from build123d import *

# Parameters (mm, degrees)
SKETCH1_R             = 75
BOSS_EXTRUDE1_DEPTH   = 10
SKETCH2_R             = 59.5
BOSS_EXTRUDE2_DEPTH   = 240
BOSS_EXTRUDE3_DEPTH   = 30
SKETCH7_R             = 10
CUT_EXTRUDE1_DEPTH    = 30
SKETCH9_R             = 4.5
CUT_EXTRUDE3_DEPTH    = 10
BODY_MOVE_COPY1_ANGLE = 90


with BuildPart() as part:
    # Sketch1 → Boss-Extrude1 (new body)
    with BuildSketch(Plane(origin=(0, 0, 0), x_dir=(1, 0, 0), z_dir=(0, 1, 0))):
        Circle(SKETCH1_R)
    extrude(amount=BOSS_EXTRUDE1_DEPTH)

    # Sketch2 → Boss-Extrude2 (add)
    with BuildSketch(Plane(origin=(0, 10, 0), x_dir=(1, 0, 0), z_dir=(0, 1, 0))):
        Circle(SKETCH2_R)
    extrude(amount=BOSS_EXTRUDE2_DEPTH)

    # Sketch6 → Boss-Extrude3 (add)
    with BuildSketch(Plane(origin=(0, 250, 0), x_dir=(1, 0, 0), z_dir=(0, 1, 0))):
        with BuildLine():
            Line((48.117044797, 35), (80, 35))
            ThreePointArc((80, 35), (101.213203436, 26.213203436), (110, 5))
            Line((110, 5), (110, -5))
            ThreePointArc((110, -5), (101.213203436, -26.213203436), (80, -35))
            Line((80, -35), (48.117044797, -35))
            ThreePointArc((48.117044797, -35), (59.5, 0), (48.117044797, 35))
        make_face()
    extrude(amount=-BOSS_EXTRUDE3_DEPTH)

    # Sketch7 → Cut-Extrude1 (cut)
    with BuildSketch(Plane(origin=(0, 250, 0), x_dir=(1, 0, 0), z_dir=(0, 1, 0))):
        Circle(SKETCH7_R)
    extrude(amount=-CUT_EXTRUDE1_DEPTH, mode=Mode.SUBTRACT)

    # Sketch9 → Cut-Extrude3 (cut)
    with BuildSketch(Plane(origin=(0, 10, 0), x_dir=(1, 0, 0), z_dir=(0, 1, 0))):
        with Locations((0, 67.096454414)):
            Circle(SKETCH9_R)
        with Locations((-67.440146023, 0)):
            Circle(SKETCH9_R)
    cut_extrude3 = extrude(amount=-CUT_EXTRUDE3_DEPTH, mode=Mode.SUBTRACT)

    # Mirror2: Cut-Extrude3 across plane
    add(cut_extrude3.mirror(Plane.XY), mode=Mode.SUBTRACT)

    # Mirror3: Cut-Extrude3 across plane
    add(cut_extrude3.mirror(Plane(origin=(0, 0, 0), x_dir=(0, 0, 1), z_dir=(1, 0, 0))), mode=Mode.SUBTRACT)


with BuildPart() as part_1:
    # Body-Move/Copy1: moved
    add(part.part.rotate(Axis((0, 0, 0), (1, 0, 0)), BODY_MOVE_COPY1_ANGLE))


solid = part_1.part
Work out the finished part from the listing and answer in its coordinate system (mm). A direction names the side the tool comes from. Coordinates: 2 decimals unless noted, no trailing zeros. Write each loop counter-clockwise with the first axis right and the second up, starting at its lowest first coordinate (ties: lowest second). Pieces come first, ordered by that corner, then holes.
1. Flat-ended cylindrical pins translate along their axes: pin 1 (10.5 mm diameter, centred on x = 0, y = 67.1, fed in from +Z); pin 2 (15 mm diameter, centred on x = 63.5, z = 228, fed in from +Y); pin 3 (7 mm diameter, centred on x = 67.44, y = 0, fed in from -Z); pin 4 (11.5 mm diameter, centred on x = 0, y = -67.1, fed in from -Z). Find the tip coordinate at first contact, or state that the pin passes through.
Results list:
pin 1: stops at z = 10
pin 2: stops at y = 35
pin 3: stops at z = 220
pin 4: stops at z = 0
2. For a pull along Y with two mould halves and no side action, classify faces 6 (the cylindrical face through (100.979, 26.445, 235.21)), 7 (the flat face through (79, 0, 220)), 8 (the cylindrical face through (-2.17, -9.76, 235.21)), 9 (the cylindrical face through (2.42, -70.89, 5.07)) as +Y half, -Y half, draft (parallel to the pull), parting line (faces both ways), or undercut.
Results list:
face 6: +Y half
face 7: draft
face 8: undercut
face 9: undercut
3. For faces 1 (the flat face through (64, 35, 235)), 2 (the flat face through (0, 0, 220)), 3 (the flat face through (64, -35, 235)), 4 (the flat face through (-34, -50, 10)), 5 (the cylindrical face through (-9.764, 74.362, 4.93)), determine the directions among +Z, -Z, +X, -X, +Y, -Y from which every point of the face is accessible in a straight line to the end or side of a thin tool.
Results list:
face 1: +Z, +X, +Y
face 2: +Z
face 3: +Z, +X, -Y
face 4: none
face 5: -Z
4. The part is cut by section A-A, the plane y = 0. Write down the section's boundary in (x, z).
Results list:
outline: (-75, 0) - (-71.94, 0) - (-71.94, 10) - (-75, 10) - close; (-62.94, 0) - (62.94, 0) - (62.94, 10) - (59.5, 10) - (59.5, 220) - (110, 220) - (110, 250) - (10, 250) - (10, 220) - (-10, 220) - (-10, 250) - (-59.5, 250) - (-59.5, 10) - (-62.94, 10) - close; (71.94, 0) - (75, 0) - (75, 10) - (71.94, 10) - close
5. The part is cut by section C-C, the plane x = 43. Write down the section's boundary in (y, z).
Results list:
outline: (-61.45, 0) - (61.45, 0) - (61.45, 10) - (41.12, 10) - (41.12, 250) - (-41.12, 250) - (-41.12, 10) - (-61.45, 10) - close
6. Consider line 1 along Y through (x, z) = (0, 3); line 2 along Y through (x, z) = (0, 241.5); line 3 along Z through (x, y) = (63.5, 26). Determine where each line is inside the solid, lowest interval first.
Results list:
line 1: y = -75 to -71.6, -62.6 to 62.6, 71.6 to 75
line 2: y = -59.5 to -10, 10 to 59.5
line 3: z = 0 to 10, 220 to 250
7. The part is cut by section B-B, the plane x = 0. Write down the section's boundary in (y, z).
Results list:
outline: (-75, 0) - (-71.6, 0) - (-71.6, 10) - (-75, 10) - close; (-62.6, 0) - (62.6, 0) - (62.6, 10) - (59.5, 10) - (59.5, 250) - (10, 250) - (10, 220) - (-10, 220) - (-10, 250) - (-59.5, 250) - (-59.5, 10) - (-62.6, 10) - close; (71.6, 0) - (75, 0) - (75, 10) - (71.6, 10) - close
8. The part is cut by section D-D, the plane z = 85.5. Write down the section's boundary in (x, y).
Results list:
outline: circle Ø119 at (0, 0)
